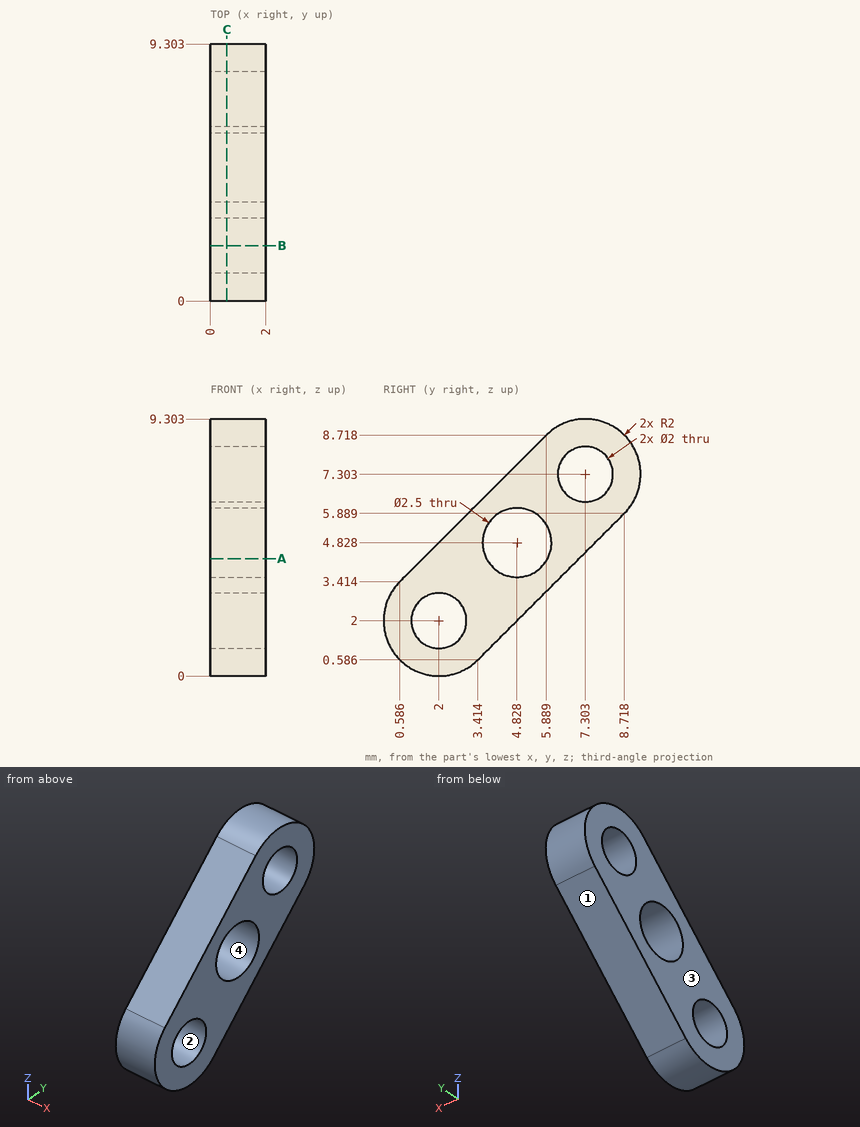
The drawing under review shows one solid part. Ordinate dimensions are in mm from its lowest x, y, z. Coordinates: 2 decimals unless noted, no trailing zeros. Order: outer loops, then holes, each group sorted by start corner. A loop starts at its lowest first (then second) coordinate and runs counter-clockwise, first axis right, second up. Notation, with made-up numbers: (-35.75, 85) -> (22.25, 85) arc R34 ccw to (22.25, 122) -> close; hole circle Ø4 at (66, 55.5). An arc over 180 degrees is marked (long way). One line per item, written item: value.
1) Draft analysis for pull direction Z (two halves, no side actions). For the marked faces 1, 2, 3 and 4, state which applies: +Z half, -Z half, draft (parallel to the pull), parting line (faces both ways), or undercut.
Output values:
face 1: -Z half
face 2: undercut
face 3: draft
face 4: undercut
2) To check wall thickness, follow probe 1 along Y at (x, z) = (0.7, 5.5) (1 decimal); probe 2 along Y at (x, z) = (0.45, 6.5) (1 decimal); probe 3 along Z at (x, y) = (1, 6.75) (1 decimal). State the ranges of each line that lie inside material, in increasing order. Write a range as [from, to].
Output values:
probe 1: y = [2.7, 3.8], [5.9, 8.3]
probe 2: y = [3.7, 6.7], [7.9, 9.1]
probe 3: z = [3.9, 6.5], [8.1, 9.2]
3) We need section B-B, the plane y = 2. Give the boundary of the cut face in (x, z).
Output values:
outline: (0, 0) -> (2, 0) -> (2, 1) -> (0, 1) -> close; (0, 3) -> (2, 3) -> (2, 4.83) -> (0, 4.83) -> close
4) We need section C-C, the plane x = 0.6. Count the separate pieces of the cut face and the enclosed holes in it.
Output values:
separate pieces: 1
enclosed holes: 3
5) We need section A-A, the plane z = 4.25. Give the boundary of the cut face in (x, y).
Output values:
outline: (0, 1.42) -> (2, 1.42) -> (2, 3.72) -> (0, 3.72) -> close; (0, 5.94) -> (2, 5.94) -> (2, 7.08) -> (0, 7.08) -> close
